Geometry: final body of the model. Coordinates: model frame, mm. Face numbers are marked on the shaded views. A direction names the side the tool comes from. Give positions to 0.01 mm unless a question says otherwise; leave off trailing zeros. Order: outer loops, then holes, each group sorted by start corner. A loop starts at its lowest first (then second) coordinate and runs counter-clockwise, first axis right, second up. Notation, with made-up numbers: (-39.5, 19) -> (-7.5, 19) arc R26 cw to (-7.5, 50) -> close; hole circle Ø3 at (-8.75, 83.25). An arc over 180 degrees is marked (long way). Write item = value, one per line.
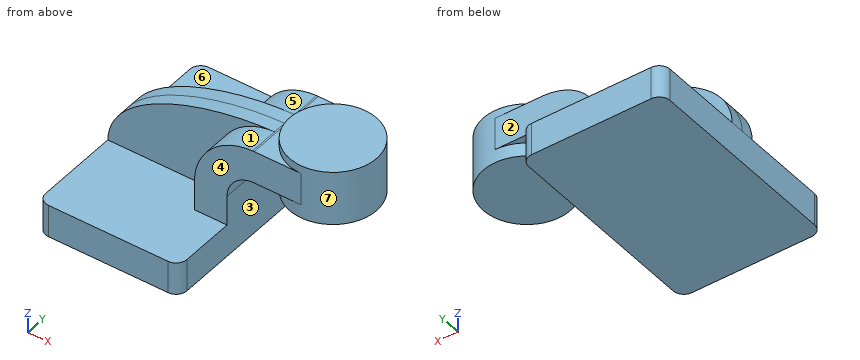
```python
from build123d import *

# Parameters (mm, degrees)
F1_DEPTH = 63.5
F2_DEPTH = 25.4
F3_DEPTH = 7.9375
F5_R     = 6.35


with BuildPart() as f1:
    # F0 (on Front) → F1 (new body, symmetric)
    with BuildSketch(Plane.XZ):
        Polygon((-41.275, -9.525), (41.275, -9.525), (41.275, 9.525), (22.225, 9.525), (-41.275, 9.525), align=None)
    extrude(amount=F1_DEPTH, both=True)

    # F0 (on Front) → F2 (join, symmetric)
    with BuildSketch(Plane.XZ):
        with BuildLine():
            Line((22.225, 9.525), (41.275, 9.525))
            Line((41.275, 9.525), (41.275, 27.0002))
            ThreePointArc((41.275, 27.0002), (45.9246798487, 38.2255201513), (57.15, 42.8752))
            Line((57.15, 42.8752), (59.0854373096, 42.8752))
            Line((59.0854373096, 42.8752), (59.0854373096, 61.9252))
            Line((59.0854373096, 61.9252), (57.15, 61.9252))
            add(Edge.make_bspline(
                [(56.190827001, 61.9120262507), (56.5119550405, 61.9175775521), (56.831694443, 61.9219686584), (57.15, 61.9252)],
                knots=[110.5788224072, 110.5788224072, 110.5788224072, 110.5788224072, 111.5045361635, 111.5045361635, 111.5045361635, 111.5045361635], degree=3))
            ThreePointArc((56.190827001, 61.9120262507), (32.1174737393, 51.3544245618), (22.225, 27.0002))
            Line((22.225, 27.0002), (22.225, 9.525))
        make_face()
        Polygon((59.0854373096, 61.9252), (59.0854373096, 42.8752), (84.4854373096, 42.8752), (84.4854373096, 50.8), (84.4854373096, 61.9252), align=None)
    extrude(amount=F2_DEPTH, both=True)

    # F0 (on Front) → F3 (join, symmetric)
    with BuildSketch(Plane.XZ):
        with BuildLine():
            add(Edge.make_bspline(
                [(-41.275, 9.525), (-40.342589198, 44.0310850968), (17.8312798934, 61.2489094196), (56.190827001, 61.9120262507)],
                knots=[0, 0, 0, 0, 110.5788224072, 110.5788224072, 110.5788224072, 110.5788224072], degree=3))
            Line((-41.275, 9.525), (22.225, 9.525))
            Line((22.225, 9.525), (22.225, 27.0002))
            ThreePointArc((22.225, 27.0002), (32.1174737393, 51.3544245618), (56.190827001, 61.9120262507))
        make_face()
    extrude(amount=F3_DEPTH, both=True)

    # F0 (on Front) → F4 (revolve)
    with BuildSketch(Plane.XZ):
        Polygon((84.4854373096, 50.8), (84.4854373096, 42.8752), (84.4854373096, 34.925), (109.8854373096, 34.925), (109.8854373096, 66.675), (84.4854373096, 66.675), (84.4854373096, 61.9252), align=None)
    revolve(axis=Axis((84.4854373096, 0, 42.8625), (0, 0, -1)))

    # F5
    f5_edges = [f1.edges().sort_by_distance(p)[0] for p in [
        (41.275, -63.5, 0),
        (-41.275, -63.5, 0),
        (41.275, 63.5, 0),
        (-41.275, 63.5, 0),
    ]]
    fillet(f5_edges, radius=F5_R)


solid = f1.part
```
1) Mould query, pull axis X, two halves, no side actions, for the marked faces 5, 6 and 7. Classes: +X half, -X half, draft (parallel to the pull), parting line (faces both ways), or undercut.
Check sheet entries:
face_5 = -X half
face_6 = draft
face_7 = undercut
2) Section query A-A (x = 76.5). Output: boundary loops of the cut face in (y, z) (3 decimals), plus the area to 3 significant figures.
Check sheet entries:
outline = (-25.4, 42.875) -> (-24.112, 42.875) -> (-24.112, 34.925) -> (24.112, 34.925) -> (24.112, 42.875) -> (25.4, 42.875) -> (25.4, 61.925) -> (24.112, 61.925) -> (24.112, 66.675) -> (-24.112, 66.675) -> (-24.112, 61.925) -> (-25.4, 61.925) -> close
area = 1,580 mm²
3) Section query B-B (y = 28). Output: boundary loops of the cut face in (x, z) (3 decimals).
Check sheet entries:
outline = (-41.275, -9.525) -> (41.275, -9.525) -> (41.275, 9.525) -> (-41.275, 9.525) -> close
4) Line query: line 1 (Z direction, x = 33, y = 38) (3 decimals); line 2 (Y direction, x = 19, z = 41); line 3 (X direction, y = 38, z = 4) (3 decimals). Output: solid intervals per line, ascending. Write a range as from..to.
Check sheet entries:
line_1 = -9.525..9.525
line_2 = -7.94..7.94
line_3 = -41.275..41.275
5) Reachability of the marked faces 1, 2, 3 and 4 from +Z, -Z, +X, -X, +Y, -Y: full face, straight path, thin tool, end or side. Return the list, or none.
Check sheet entries:
face_1 = +Z, -X, -Y
face_2 = +Z, +X, -X, +Y
face_3 = -Z, +X, +Y, -Y
face_4 = +Z, +X, -X, -Y
6) First-contact query: P1, Ø2, axis at x = 29.5, z = 39.5, coming from the -Y side; P2, Ø15.5, axis at x = 50.5, z = 40.5, coming from the +Y side; P3, Ø3, axis at x = -3.5, y = -8.5, coming from the +Z side. Flat tips, straight axial feed; report the tip coordinate or a pass-through.
Check sheet entries:
P1 = -25.4
P2 = 25.4
P3 = 50.3
